The model under review builds one solid part; all positions refer to its coordinate system, in mm. Coordinates: 2 decimals unless noted, no trailing zeros. Order: outer loops, then holes, each group sorted by start corner. A loop starts at its lowest first (then second) coordinate and runs counter-clockwise, first axis right, second up. Notation, with made-up numbers: (-26, -35) -> (-19, -35) arc R25 cw to (-19, 1) -> close; hole circle Ø6 at (70.5, 13). An arc over 180 degrees is marked (long way). Use one line per item in the form item = value. Start each with the question number.
(1) Wall thickness on line 1 along Z through (x, y) = (114.3, -2.7); line 2 along X through (y, z) = (-2.65, 11); line 3 along Z through (x, y) = (76.2, -1.15): over which ranges is each line inside the solid? List them lowest first.
(2) Take a section at D-D (x = 69.85). State the section outline as (y, z) points, then the cut area to 3 significant figures.
(3) Mouldability with a two-part tool opening along X and no side actions: class faces 1 (the flat face through (127, -2, 19)), 2 (the cylindrical face through (84.935, -1.972, 13.451)), 3 (the cylindrical face through (65.028, -2.028, 49.351)), 4 (the flat face through (112, -2, 38.1)) as +X half, -X half, draft (parallel to the pull), parting line (faces both ways), or undercut.
(4) Insertion check: pin 1 Ø2 at (x, y) = (112, -2.5) entering from +Z; pin 2 Ø1 at (x, y) = (78.5, -3.5) entering from +Z. Each pin has a flat end and moves straight along its axis. Give the tip position at first contact, or say it passes through.
(5) Take a section at A-A (z = 6.35). State the section outline as (x, y) points, then the cut area to 3 significant figures.
(6) Take a section at C-C (y = -1.95). State the section outline as (x, z) points.
(7) Take a section at B-B (x = 114.3). State the section outline as (y, z) points, then the cut area to 3 significant figures.
```python
from build123d import *

# Parameters (mm, degrees)
SKETCH1_R           = 2.5
BOSS_EXTRUDE1_DEPTH = 4
FILLET1_R           = 5.08


with BuildPart() as part:
    # Sketch1 → Boss-Extrude1 (new body)
    with BuildSketch(Plane.XZ):
        Polygon((127, 38.1), (101.6, 38.1), (76.2, 50.8), (63.5, 50.8), (63.5, 0), (127, 0), align=None)
        with Locations((69.85, 12.7)):
            Circle(SKETCH1_R, mode=Mode.SUBTRACT)
        with Locations((82.55, 12.7)):
            Circle(SKETCH1_R, mode=Mode.SUBTRACT)
        with Locations((114.3, 6.35)):
            Circle(SKETCH1_R, mode=Mode.SUBTRACT)
        with Locations((95.25, 12.7)):
            Circle(SKETCH1_R, mode=Mode.SUBTRACT)
        with Locations((114.3, 25.4)):
            Circle(SKETCH1_R, mode=Mode.SUBTRACT)
        with Locations((76.2, 38.1)):
            Circle(SKETCH1_R, mode=Mode.SUBTRACT)
    extrude(amount=BOSS_EXTRUDE1_DEPTH)

    # Fillet1
    fillet1_edges = [part.edges().sort_by_distance(p)[0] for p in [
        (63.5, -2, 50.8),
        (76.2, -2, 50.8),
        (101.6, -2, 38.1),
        (127, -2, 38.1),
        (127, -2, 0),
        (63.5, -2, 0),
    ]]
    fillet(fillet1_edges, radius=FILLET1_R)


solid = part.part
```
Findings:
q1.line_1 = 0 to 3.85, 8.85 to 22.9, 27.9 to 38.1
q1.line_2 = 63.5 to 68.02, 71.68 to 80.72, 84.38 to 93.42, 97.08 to 127
q1.line_3 = 0 to 35.6, 40.6 to 50.66
q2.outline = (-4, 0) -> (0, 0) -> (0, 10.2) -> (-4, 10.2) -> close; (-4, 15.2) -> (0, 15.2) -> (0, 50.8) -> (-4, 50.8) -> close
q2.area = 183 mm²
q3.face_1 = +X half
q3.face_2 = undercut
q3.face_3 = -X half
q3.face_4 = draft
q4.pin_1 = 38.1
q4.pin_2 = 49.9
q5.outline = (63.5, -4) -> (111.8, -4) -> (111.8, 0) -> (63.5, 0) -> close; (116.8, -4) -> (127, -4) -> (127, 0) -> (116.8, 0) -> close
q5.area = 234 mm²
q6.outline = (63.5, 5.08) arc R5.08 ccw to (68.58, 0) -> (121.92, 0) arc R5.08 ccw to (127, 5.08) -> (127, 33.02) arc R5.08 ccw to (121.92, 38.1) -> (102.8, 38.1) arc R5.08 cw to (100.53, 38.64) -> (77.27, 50.26) arc R5.08 ccw to (75, 50.8) -> (68.58, 50.8) arc R5.08 ccw to (63.5, 45.72) -> close; hole circle Ø5 at (69.85, 12.7); hole circle Ø5 at (76.2, 38.1); hole circle Ø5 at (82.55, 12.7); hole circle Ø5 at (95.25, 12.7); hole circle Ø5 at (114.3, 6.35); hole circle Ø5 at (114.3, 25.4)
q7.outline = (-4, 0) -> (0, 0) -> (0, 3.85) -> (-4, 3.85) -> close; (-4, 8.85) -> (0, 8.85) -> (0, 22.9) -> (-4, 22.9) -> close; (-4, 27.9) -> (0, 27.9) -> (0, 38.1) -> (-4, 38.1) -> close
q7.area = 112 mm²
